Verification items for the finished model (mm, model axes). Face numbers are marked on the shaded views. A direction names the side the tool comes from. Round coordinates to 2 decimals unless told otherwise and drop trailing zeros. Loops run counter-clockwise (first coordinate to the right, second up) from the corner with the lowest first, then second, coordinate; pieces in that order, holes last. Notation, with made-up numbers: (-3.5, -31) -> (51.5, -31) arc R20 cw to (51.5, -24) -> close; hole circle Ø1 at (-24, -35.5). An arc over 180 degrees is marked (long way). Use a Markdown table: item, result. Add a question column.
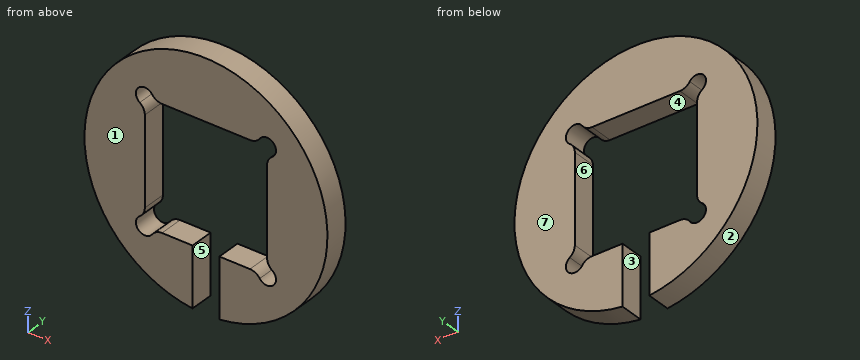
```python
from build123d import *

# Parameters (mm, degrees)
BOSS_EXTRUDE1_DEPTH = 4
FILLET1_R           = 2


with BuildPart() as part:
    # Sketch1 → Boss-Extrude1 (new body)
    with BuildSketch(Plane(origin=(0, 0, 0), x_dir=(1, 0, 0), z_dir=(0, 1, 0))):
        with BuildLine():
            ThreePointArc((1.5, 0), (-1.060660172, -1.060660172), (0, 1.5))
            Line((0, 1.5), (0, 19))
            ThreePointArc((0, 19), (-1.060660172, 21.560660172), (1.5, 20.5))
            Line((1.5, 20.5), (8, 20.5))
            Line((8, 20.5), (8, 30.5))
            ThreePointArc((8, 30.5), (10.25, -10.124616561), (12.5, 30.5))
            Line((12.5, 30.5), (12.5, 20.5))
            Line((12.5, 20.5), (19, 20.5))
            ThreePointArc((19, 20.5), (21.560660172, 21.560660172), (20.5, 19))
            Line((20.5, 19), (20.5, 1.5))
            ThreePointArc((20.5, 1.5), (21.560660172, -1.060660172), (19, 0))
            Line((19, 0), (1.5, 0))
        make_face()
    extrude(amount=BOSS_EXTRUDE1_DEPTH)

    # Fillet1
    fillet1_edges = [part.edges().sort_by_distance(p)[0] for p in [
        (0, 2, -19),
        (0, 2, -1.5),
        (1.5, 2, 0),
        (19, 2, 0),
        (20.5, 2, -1.5),
        (20.5, 2, -19),
        (19, 2, -20.5),
        (1.5, 2, -20.5),
    ]]
    fillet(fillet1_edges, radius=FILLET1_R)


solid = part.part
```
1) Access from +Z, -Z, +X, -X, +Y, -Y to the whole of each face (thin tool, end or side, straight path). Record for the marked faces 5, 6 and 7.
2) Go/stop test with flat-tipped pins: pin 1 (1 mm diameter, centred on x = -0.5, y = 0.5, fed in from -Z); pin 2 (2 mm diameter, centred on x = 5, y = 2.5, fed in from +Z); pin 3 (2 mm diameter, centred on y = 3, z = -5.5, fed in from -X). Record where each tip stops, or that it passes through.
3) Release check for a two-part mould opening along X. For the marked faces 1, 2, 3 and 4 record: released by +X, released by -X, zero draft, split by the parting line, or undercut.
4) Thickness scan on line 1 (X direction, y = 0.95, z = 1); line 2 (Z direction, x = 13, y = 1.5); line 3 (X direction, y = 3.8, z = -27). Record the ranges inside material, lowest first.
5) Sectioned sample at B-B on z = -28. Enter the section's corners in (x, y), then the cut area to 3 significant figures.
6) Sectioned sample at D-D on z = -7.5. Enter the section's corners in (x, y), then the cut area to 3 significant figures.
7) Sectioned sample at C-C on x = 10.25. Enter the section's corners in (y, z), then the cut area to 3 significant figures.
8) Sectioned sample at A-A on y = 3. Enter the section's corners in (x, z), then the cut area to 3 significant figures.
Geometry results:
| question | item | result |
|---|---|---|
| 1 | face 5 | -Z, +Y, -Y |
| 1 | face 6 | +Y, -Y |
| 1 | face 7 | +Z, -Z, +X, -X, +Y |
| 2 | pin 1 | z = -27.86 |
| 2 | pin 2 | z = 9.68 |
| 2 | pin 3 | x = -9.78 |
| 3 | face 1 | zero draft |
| 3 | face 2 | split by the parting line |
| 3 | face 3 | undercut |
| 3 | face 4 | undercut |
| 4 | line 1 | -6.74 to -1.12, 1.12 to 19.38, 21.62 to 27.24 |
| 4 | line 2 | -30.44 to -20.5, 0 to 9.94 |
| 4 | line 3 | -1.35 to 8, 12.5 to 21.85 |
| 5 | outline | (0.25, 0) -> (8, 0) -> (8, 4) -> (0.25, 4) -> close; (12.5, 0) -> (20.25, 0) -> (20.25, 4) -> (12.5, 4) -> close |
| 5 | area | 62.0 mm^2 |
| 6 | outline | (-9.94, 0) -> (0, 0) -> (0, 4) -> (-9.94, 4) -> close; (20.5, 0) -> (30.44, 0) -> (30.44, 4) -> (20.5, 4) -> close |
| 6 | area | 79.5 mm^2 |
| 7 | outline | (0, 0) -> (4, 0) -> (4, 10.12) -> (0, 10.12) -> close |
| 7 | area | 40.5 mm^2 |
| 8 | outline | (-0.86, -19.27) arc R2 ccw to (0, -17.63) -> (0, -2.87) arc R2 ccw to (-0.86, -1.23) arc R1.5 cw (long way) to (1.23, 0.86) arc R2 ccw to (2.87, 0) -> (17.63, 0) arc R2 ccw to (19.27, 0.86) arc R1.5 cw (long way) to (21.36, -1.23) arc R2 ccw to (20.5, -2.87) -> (20.5, -17.63) arc R2 ccw to (21.36, -19.27) arc R1.5 cw (long way) to (19.27, -21.36) arc R2 ccw to (17.63, -20.5) -> (12.5, -20.5) -> (12.5, -30.5) arc R20.37 ccw (long way) to (8, -30.5) -> (8, -20.5) -> (2.87, -20.5) arc R2 ccw to (1.23, -21.36) arc R1.5 cw (long way) to start |
| 8 | area | 815 mm^2 |
